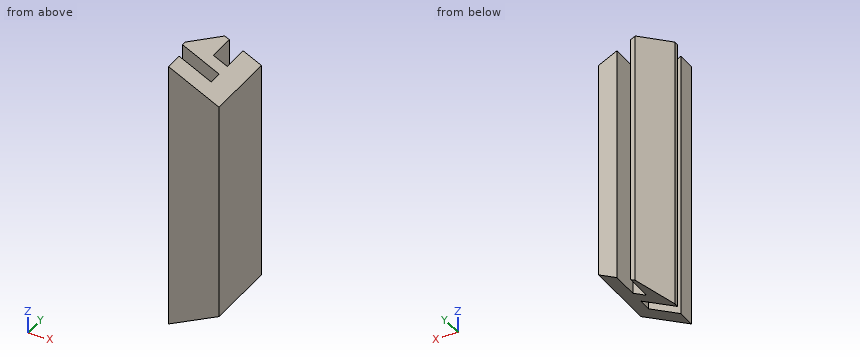
```python
from build123d import *

# Parameters (mm, degrees)
DODANIE_WYCI_GNI_CIE1_DEPTH = 70
SZKIC2_OUTSIDE_W            = 28.56
SZKIC2_OUTSIDE_H            = 86.56
WYTNIJ_WYCI_GNI_CIE1_DEPTH  = 73.249567473


with BuildPart() as part:
    # Szkic1 → Dodanie-wyciągnięcie1 (new body)
    with BuildSketch(Plane.XY):
        Polygon((0, 0), (-7, 0), (-7, -4), (-0.506849315, -4), (4, -4), (4, 12), (0, 12), (0, 6), (-3, 6), (-3, 12), (-4, 12), (-8, 4), (-8, 3), (0, 3), align=None)
    extrude(amount=DODANIE_WYCI_GNI_CIE1_DEPTH)

    # Szkic2 outside → Wytnij-wyciągnięcie1 (cut, through all)
    with BuildSketch(Plane(origin=(0, 12, 0), x_dir=(1, 0, 0), z_dir=(0, 1, 0))):
        with Locations((-2, -35)):
            Rectangle(SZKIC2_OUTSIDE_W, SZKIC2_OUTSIDE_H)
        Polygon((-15.924171966, -0.266842792), (4, -10.231080013), (4, -58.231080013), (-15.924171966, -68.195317233), align=None, mode=Mode.SUBTRACT)
    extrude(amount=-WYTNIJ_WYCI_GNI_CIE1_DEPTH, mode=Mode.SUBTRACT)


solid = part.part
```
Read the model definition and answer for the solid it produces. Units are mm, in the model's axes. Round coordinates to 2 decimals unless told otherwise and drop trailing zeros. Loops run counter-clockwise (first coordinate to the right, second up) from the corner with the lowest first, then second, coordinate; pieces in that order, holes last. Notation, with made-up numbers: (14.25, 9) -> (35.25, 9) arc R13 cw to (35.25, 24) -> close; hole circle Ø11 at (-36, 67.5). An arc over 180 degrees is marked (long way). One line per item, written item: value.
1) A cutting plane is placed at B-B (x = -2). Determine the outline of the cut face in (y, z).
Answer list:
outline: (-4, 7.23) -> (0, 7.23) -> (0, 61.23) -> (-4, 61.23) -> close; (3, 7.23) -> (6, 7.23) -> (6, 61.23) -> (3, 61.23) -> close
2) A cutting plane is placed at D-D (y = -0.75). Determine the outline of the cut face in (x, z), and give its area (3 significant figures).
Answer list:
outline: (-7, 4.73) -> (4, 10.23) -> (4, 58.23) -> (-7, 63.73) -> close
area: 589 mm²
3) Consider L1, parallel to Y at x = -3.5, z = 60; L2, parallel to Y at x = -2.25, z = 24.5; L3, parallel to X at y = -1, z = 18. Determine where each line is inside the solid, lowest interval first. Write a range as [from, to].
Answer list:
L1: y = [-4, 0], [3, 12]
L2: y = [-4, 0], [3, 6]
L3: x = [-7, 4]
4) Flat-ended cylindrical pins translate along their axes: P1, Ø5, axis at y = 8, z = 44, coming from the -X side; P2, Ø6, axis at x = -3, y = 5, coming from the -Z side; P3, Ø1.5, axis at x = -1, z = 26, coming from the +Y side. Find the tip coordinate at first contact, or state that the pin passes through.
Answer list:
P1: stops at x = -7.25
P2: stops at z = 5.23
P3: stops at y = 6
5) A cutting plane is placed at A-A (y = 9). Determine the outline of the cut face in (x, z).
Answer list:
outline: (-5.5, 5.48) -> (-3, 6.73) -> (-3, 61.73) -> (-5.5, 62.98) -> close; (0, 8.23) -> (4, 10.23) -> (4, 58.23) -> (0, 60.23) -> close
6) A cutting plane is placed at C-C (z = 14). Determine the outline of the cut face in (x, y).
Answer list:
outline: (-8, 3) -> (0, 3) -> (0, 0) -> (-7, 0) -> (-7, -4) -> (4, -4) -> (4, 12) -> (0, 12) -> (0, 6) -> (-3, 6) -> (-3, 12) -> (-4, 12) -> (-8, 4) -> close
